Check sheet for the drawn part. Datum: minimum x, y, z corner. Units: mm. A direction names the side the tool comes from. Give positions to 0.01 mm unless a question says otherwise; leave off trailing zeros. Order: outer loops, then holes, each group sorted by start corner. A loop starts at its lowest first (then second) coordinate and runs counter-clockwise, first axis right, second up. Notation, with made-up numbers: M -13,-40 L -5,-40 A31 ccw -5,-4 Z; hole C -21.5,-12 d3. An arc over 180 degrees is marked long. Put each result on its own line as item: value. Start each with the question number.
Q1. Go/stop test with flat-tipped pins: pin 1 (4.5 mm diameter, centred on x = 42.22, y = 145.14, fed in from +Z); pin 2 (1.5 mm diameter, centred on x = 9.5, z = 4, fed in from +Y) (3 decimals); pin 3 (2 mm diameter, centred on y = 30, z = 7, fed in from -X); pin 4 (3 mm diameter, centred on y = 46.5, z = 3.5, fed in from -X). Record where each tip stops, or that it passes through.
Q2. Section check A-A on x = 42.22. Record the cut outline in (y, z) (3 decimals), then the cut area to 3 significant figures.
Q3. Access from +Z, -Z, +X, -X, +Y, -Y to the whole of each face (thin tool, end or side, straight path). Record for the marked faces 1 and 2.
Q4. Material ranges on L1, parallel to Z at x = 44, y = 146.5; L2, parallel to Y at x = 33.5, z = 3.25 (3 decimals); L3, parallel to X at y = 125, z = 6.5 (3 decimals), recorded low to high.
Q5. Section check B-B on z = 8. Record the cut outline in (x, y) (3 decimals), then the cut area to 3 significant figures.
Q6. Section check D-D on y = 127. Record the cut outline in (x, z).
Q7. Section check C-C on y = 81. Record the cut outline in (x, z), then the cut area to 3 significant figures.
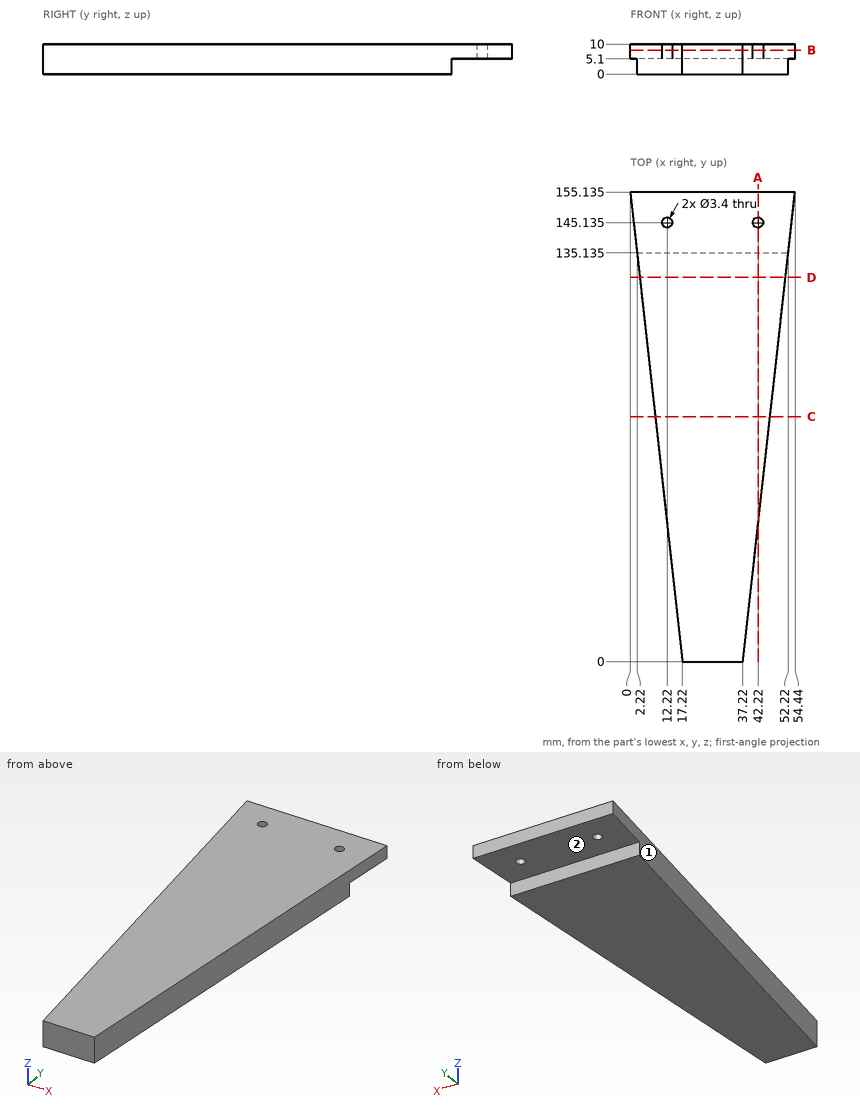
Results found:
1. pin 1: stops at z = 10
1. pin 2: stops at y = 135.135
1. pin 3: stops at x = 13.78
1. pin 4: stops at x = 11.89
2. outline: M 45.045,0 L 135.135,0 L 135.135,5.1 L 143.435,5.1 L 143.435,10 L 45.045,10 Z; M 146.835,5.1 L 155.135,5.1 L 155.135,10 L 146.835,10 Z
2. area: 982 mm^2
3. face 1: +Z, -Z, -X, -Y
3. face 2: -Z, +X, -X, +Y
4. L1: z = 5.1 to 10
4. L2: y = 0 to 135.135
4. L3: x = 3.345 to 51.095
5. outline: M 0,155.135 L 17.22,0 L 37.22,0 L 54.44,155.135 Z; hole C 12.22,145.135 d3.4; hole C 42.22,145.135 d3.4
5. area: 5,760 mm^2
6. outline: M 3.12,0 L 51.32,0 L 51.32,10 L 3.12,10 Z
7. outline: M 8.23,0 L 46.21,0 L 46.21,10 L 8.23,10 Z
7. area: 380 mm^2
